Read the model definition and answer for the solid it produces. Units are mm, in the model's axes. A direction names the side the tool comes from. Round coordinates to 2 decimals unless told otherwise and drop trailing zeros. Write each loop counter-clockwise with the first axis right and the second up, starting at its lowest first coordinate (ties: lowest second). Pieces come first, ordered by that corner, then holes. Notation, with made-up numbers: M 12.5,36.25 L 53.5,36.25 A6 ccw 53.5,45.25 Z; hole C 55,-3.5 d1. An arc over 180 degrees is marked long. Use one line per item in the form item = value. Start each with the question number.
```python
from build123d import *

# Parameters (mm, degrees)
REVOLVE1_ANGLE           = 75
REVOLVE1_OTHER_WAY_ANGLE = 75
BOSS_EXTRUDE3_START      = -12
BOSS_EXTRUDE3_OUTLINE_R  = 6
BOSS_EXTRUDE3_DEPTH      = 12
CUT_EXTRUDE1_DEPTH       = 10
CUT_EXTRUDE2_DEPTH       = 21


# Read off the part's stored shape, not the designer's step: Boss-Extrude3
with BuildPart() as part:
    # Sketch1 → Revolve1 (revolve)
    with BuildSketch(Plane.XY):
        Polygon((-6, -8), (-6, -6), (5, -6), (5, -9.845299462), (3, -11), (3, -31.845299462), (5, -33), (5, -36), (-5, -36), (-5, -33), (-3, -31.845299462), (-3, -11), (-5, -9.845299462), (-5, -8), align=None)
    revolve(axis=Axis((0, 0, 0), (1, 0, 0)), revolution_arc=REVOLVE1_ANGLE)

    # Sketch1 → Revolve1 other way (revolve)
    with BuildSketch(Plane.XY):
        Polygon((-6, -8), (-6, -6), (5, -6), (5, -9.845299462), (3, -11), (3, -31.845299462), (5, -33), (5, -36), (-5, -36), (-5, -33), (-3, -31.845299462), (-3, -11), (-5, -9.845299462), (-5, -8), align=None)
    revolve(axis=Axis((0, 0, 0), (-1, 0, 0)), revolution_arc=REVOLVE1_OTHER_WAY_ANGLE)

    # Boss-Extrude3 outline → Boss-Extrude3 (add)
    with BuildSketch(Plane.ZY.offset(6).offset(BOSS_EXTRUDE3_START)):
        with BuildLine():
            ThreePointArc((-5.795554958, -1.552914271), (0, 6), (5.795554958, -1.552914271))
            Line((5.795554958, -1.552914271), (13.589907909, -3.641404849))
            ThreePointArc((13.589907909, -3.641404849), (11.451770728, -2.21274726), (10.625184089, 0.222298456))
            Line((10.625184089, 0.222298456), (10.625184089, 22.4840758))
            ThreePointArc((10.625184089, 22.4840758), (10.449472793, 23.656601242), (9.937776134, 24.726113701))
            ThreePointArc((9.937776134, 24.726113701), (0, 30), (-9.937776134, 24.726113701))
            ThreePointArc((-9.937776134, 24.726113701), (-10.449472793, 23.656601242), (-10.625184089, 22.4840758))
            Line((-10.625184089, 22.4840758), (-10.625184089, 0.222298456))
            ThreePointArc((-10.625184089, 0.222298456), (-11.451770728, -2.21274726), (-13.589907909, -3.641404849))
            Line((-13.589907909, -3.641404849), (-5.795554958, -1.552914271))
        make_face()
        with Locations((0, 18)):
            Circle(BOSS_EXTRUDE3_OUTLINE_R, mode=Mode.SUBTRACT)
    extrude(amount=BOSS_EXTRUDE3_DEPTH)

    # Sketch4 → Cut-Extrude1 (cut)
    with BuildSketch(Plane(origin=(0, 0, 0), x_dir=(1, 0, 0), z_dir=(0, -0.9659258262890691, 0.258819045102518))):
        Polygon((-3, -14.069307952), (-3, -11), (-5, -9.845299462), (-5, -8), (-6, -8), (-6, -14.069307952), align=None)
    extrude(amount=-CUT_EXTRUDE1_DEPTH, mode=Mode.SUBTRACT)

    # Sketch5 → Cut-Extrude2 (cut)
    with BuildSketch(Plane(origin=(0, 0, 0), x_dir=(1, 0, 0), z_dir=(0, -0.9659258262890691, -0.25881904510251813))):
        Polygon((-3, 14.069307952), (-3, 11), (-5, 9.845299462), (-5, 8), (-6, 8), (-6, 14.069307952), align=None)
    extrude(amount=-CUT_EXTRUDE2_DEPTH, mode=Mode.SUBTRACT)


solid = part.part
```
Q1. For a pull along Y with two mould halves and no side action, classify faces 1 (the face through (-3, -16, 2)), 2 (the face through (5, -34, 0)), 3 (the face through (0.084, 23.641, 10.454)) as +Y half, -Y half, draft (parallel to the pull), parting line (faces both ways), or undercut.
Q2. Find section B-B on y = 18. Write down the section's boundary in (x, z).
Q3. Each of these flat-tipped pins is pushed along its axis until it touches: pin 1 Ø3.5 at (x, y) = (-0.5, 14.5) entering from +Z; pin 2 Ø8.5 at (y, z) = (-21, -2) entering from +X; pin 3 Ø4 at (x, z) = (0.5, -20) entering from -Y. Where does it stop, or does it pass through?
Q4. A tool of negligible diameter and unlimited length cuts with its end or side. For faces 4 (the face through (-5.5, -8, -0.1)), 5 (the face through (-5, -33.4, 0.2)), 6 (the face through (0, 11, 10.625)), 7 (the face through (-4.21, -1.54, -10.25)), 8 (the face through (3.35, -32.04, -0.59)), from which of +Z, -Z, +X, -X, +Y, -Y can it reach the whole face along a straight path? Write none if from no direction.
Q5. Straight lines are drawn through the part: line 1 (Z direction, x = 2.5, y = 0); line 2 (Y direction, x = -3.5, z = -3.5); line 3 (X direction, y = -27, z = 6). For each, find the intervals that lie inside material, in ascending order. Write a range as [from, to].
Q6. Find section C-C on x = 4. Write down the section's boundary in (y, z), and give its area (3 significant figures).
Q7. Find section A-A on z = 0. Write down the section's boundary in (x, y), and give its area (3 significant figures).
Response:
q1.face_1 = undercut
q1.face_2 = draft
q1.face_3 = +Y half
q2.outline = M -6,-10.63 L 6,-10.63 L 6,-6 L -6,-6 Z; M -6,6 L 6,6 L 6,10.63 L -6,10.63 Z
q3.pin_1 = 10.63
q3.pin_2 = 3
q3.pin_3 = -31.18
q4.face_4 = -X, -Y
q4.face_5 = +Z, -Z, -X, -Y
q4.face_6 = +Z, +X, -X, +Y
q4.face_7 = -Z, -X
q4.face_8 = +X
q5.line_1 = [-10.63, -6], [6, 10.63]
q5.line_2 = [-35.83, -31.94], [-10.12, -4.87], [4.87, 13.13], [22.87, 29.48]
q5.line_3 = [-3, 3]
q6.outline = M -9.32,-34.77 L -8.39,-31.32 A32.42 cw -8.39,31.32 L -9.32,34.77 A36 ccw Z; M -3.64,-13.59 A4 cw 0.22,-10.63 L 22.48,-10.63 A4 ccw 24.73,-9.94 A12 ccw 24.73,9.94 A4 ccw 22.48,10.63 L 0.22,10.63 A4 cw -3.64,13.59 L -2.7,10.07 A10.42 ccw -2.7,-10.07 Z; hole C 0,0 d12; hole C 18,0 d12
q6.area = 868 mm²
q7.outline = M -6,-8 L -5,-8 L -5,-9.85 L -3,-11 L -3,-31.85 L -5,-33 L -5,-36 L 5,-36 L 5,-33 L 3,-31.85 L 3,-11 L 5,-9.85 L 5,-6 L -6,-6 Z; M -6,6 L 6,6 L 6,12 L -6,12 Z; M -6,24 L 6,24 L 6,30 L -6,30 Z
q7.area = 358 mm²
